from build123d import *

# Parameters (mm, degrees)
F0_W     = 1800
F0_H     = 450
F1_DEPTH = 20
F2_W     = 20
F2_H     = 450
F3_DEPTH = 400
F4_W     = 1780
F4_H     = 450
F4_W_2   = 20
F5_DEPTH = 20
F6_W     = 400
F6_H     = 20
F7_DEPTH = 660


with BuildPart() as f1:
    # F0 (on Top) → F1 (new body)
    with BuildSketch(Plane.XY):
        Rectangle(F0_W, F0_H)
    extrude(amount=F1_DEPTH)

    # F2 (on face) → F3 (join)
    with BuildSketch(Plane.XY.offset(20)):
        with Locations((-890, 0)):
            Rectangle(F2_W, F2_H)
        with Locations((890, 0)):
            Rectangle(F2_W, F2_H)
        with Locations((340, 0)):
            Rectangle(F2_W, F2_H)
        with Locations((-340, 0)):
            Rectangle(F2_W, F2_H)
    extrude(amount=F3_DEPTH)

    # F4 (on face) → F5 (join)
    with BuildSketch(Plane.XY.offset(420)):
        with Locations((-10, 0)):
            Rectangle(F4_W, F4_H)
        with Locations((890, 0)):
            Rectangle(F4_W_2, F4_H)
    extrude(amount=F5_DEPTH)

    # F6 (on face) → F7 (join)
    with BuildSketch(Plane.YZ.offset(-330)):
        with Locations((25, 150)):
            Rectangle(F6_W, F6_H)
        with Locations((25, 290)):
            Rectangle(F6_W, F6_H)
    extrude(amount=F7_DEPTH)


solid = f1.part
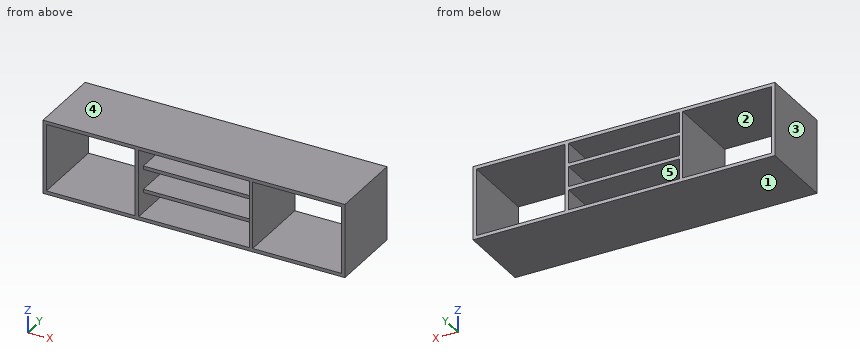
Can you work these out from the model? Positions are in its coordinate system, mm. Face numbers are marked on the shaded views. A direction names the side the tool comes from. Round coordinates to 2 decimals unless told otherwise and drop trailing zeros. Write each loop counter-clockwise with the first axis right and the second up, starting at its lowest first coordinate (ties: lowest second). Pieces come first, ordered by that corner, then holes. Notation, with made-up numbers: M 13,12.5 L 62,12.5 A20 cw 62,17.5 Z; hole C 49.25,-15.75 d11. An arc over 180 degrees is marked long. Use CSV: the item, a comma, the result in double quotes.
(1) We'd pull the mould along Z, two halves only. Please class the marked faces 3, 4 and 5: +Z half, -Z half, draft (parallel to the pull), parting line (faces both ways), or undercut.
Check values:
face 3,"draft"
face 4,"+Z half"
face 5,"undercut"
(2) Imagine slicing it at D-D (x = 170). Write out the boundary of the cut face in (y, z), plus the area to 3 significant figures.
Check values:
outline,"M -225,0 L 225,0 L 225,20 L -225,20 Z; M -225,420 L 225,420 L 225,440 L -225,440 Z; M -175,140 L 225,140 L 225,160 L -175,160 Z; M -175,280 L 225,280 L 225,300 L -175,300 Z"
area,"34,000 mm^2"
(3) I'm going to push flat-ended pins straight in: pin 1 (6 mm diameter, centred on x = 64, z = 286, fed in from -Y); pin 2 (2 mm diameter, centred on x = 263.5, y = 69, fed in from -Z). Where does each tip first touch, or does it pass through?
Check values:
pin 1,"y = -175"
pin 2,"z = 0"
(4) Imagine slicing it at C-C (y = 18). Write out the boundary of the cut face in (x, z).
Check values:
outline,"M -900,0 L 900,0 L 900,440 L -900,440 Z; hole M -880,20 L -350,20 L -350,420 L -880,420 Z; hole M -330,20 L 330,20 L 330,140 L -330,140 Z; hole M -330,160 L 330,160 L 330,280 L -330,280 Z; hole M -330,300 L 330,300 L 330,420 L -330,420 Z; hole M 350,20 L 880,20 L 880,420 L 350,420 Z"
(5) I need wall thicknesses on line 1 along X through (y, z) = (-95, 333.5); line 2 along X through (y, z) = (23, 155); line 3 along Z through (x, y) = (-62, -117). Which ranges of each line are inside material? Lowest first, please.
Check values:
line 1,"-900 to -880, -350 to -330, 330 to 350, 880 to 900"
line 2,"-900 to -880, -350 to 350, 880 to 900"
line 3,"0 to 20, 140 to 160, 280 to 300, 420 to 440"
(6) Imagine slicing it at B-B (x = 691). Write out the boundary of the cut face in (y, z), plus the area to 3 significant figures.
Check values:
outline,"M -225,0 L 225,0 L 225,20 L -225,20 Z; M -225,420 L 225,420 L 225,440 L -225,440 Z"
area,"18,000 mm^2"
(7) Imagine slicing it at A-A (z = 72.5). Write out the boundary of the cut face in (x, y), plus the area to 3 significant figures.
Check values:
outline,"M -900,-225 L -880,-225 L -880,225 L -900,225 Z; M -350,-225 L -330,-225 L -330,225 L -350,225 Z; M 330,-225 L 350,-225 L 350,225 L 330,225 Z; M 880,-225 L 900,-225 L 900,225 L 880,225 Z"
area,"36,000 mm^2"
(8) On a 3-axis mill with a long thin cutter (end or side, diameter ignored), from which of +Z, -Z, +X, -X, +Y, -Y can I reach the whole of each face in a straight line? I mean the marked faces 1 and 2. Say none if no direction works.
Check values:
face 1,"-Z, +X, -X, +Y, -Y"
face 2,"+Y, -Y"
